Part model, mm, in its own coordinate system. Round coordinates to 2 decimals unless told otherwise and drop trailing zeros. Write each loop counter-clockwise with the first axis right and the second up, starting at its lowest first coordinate (ties: lowest second). Pieces come first, ordered by that corner, then holes. Notation, with made-up numbers: M 24,65 L 82,65 A22 cw 82,99 Z; hole C -35.5,-30.75 d11. An arc over 180 degrees is marked long. Use one line per item in the form item = value. Start each with the question number.
Item 1: Cut at A-A, the plane x = -29. Give the cut face in (y, z).
Item 2: Probe L1, parallel to X at y = -6.25, z = 24.5; L2, parallel to X at y = -11.25, z = -23.5. List the from-to ranges inside material, lowest first.
Item 3: Cut at B-B, the plane z = 24.5. Give the cut face in (x, y), then the cut area to 3 significant figures.
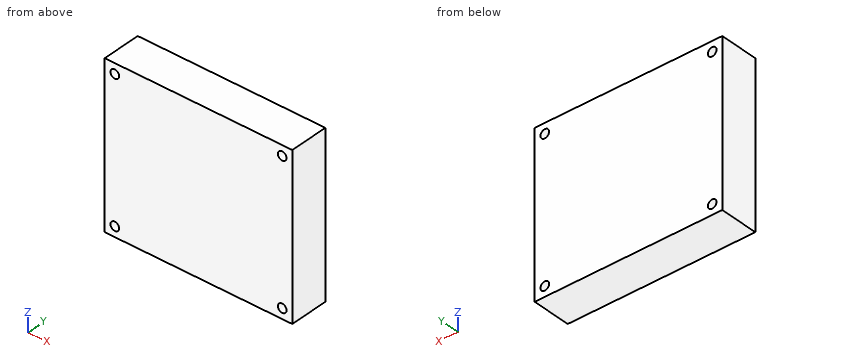
from build123d import *

# Parameters (mm, degrees)
SKETCH1_W           = 65
SKETCH1_H           = 56
BOSS_EXTRUDE1_DEPTH = 13.4
CUT_EXTRUDE1_REACH  = 46.942
SKETCH2_R           = 1.5


with BuildPart() as part:
    # Sketch1 → Boss-Extrude1 (new body)
    with BuildSketch(Plane(origin=(0, 0, 0), x_dir=(1, 0, 0), z_dir=(0, 1, 0))):
        Rectangle(SKETCH1_W, SKETCH1_H)
    extrude(amount=-BOSS_EXTRUDE1_DEPTH)

    # Sketch2 → Cut-Extrude1 (cut, up to next)
    with BuildSketch(Plane(origin=(0, 0, 0), x_dir=(1, 0, 0), z_dir=(0, 1, 0)), mode=Mode.PRIVATE) as cut_extrude1_sk1:
        with Locations(Location((29, 24.5, 0), (0, 0, 270))):
            Circle(SKETCH2_R)
    cut_extrude1_tool1 = extrude(cut_extrude1_sk1.sketch, amount=-CUT_EXTRUDE1_REACH, mode=Mode.PRIVATE) & part.part
    # Sketch2 → Cut-Extrude1 (cut, up to next)
    with BuildSketch(Plane(origin=(0, 0, 0), x_dir=(1, 0, 0), z_dir=(0, 1, 0)), mode=Mode.PRIVATE) as cut_extrude1_sk2:
        with Locations(Location((29, -24.5, 0), (0, 0, 270))):
            Circle(SKETCH2_R)
    cut_extrude1_tool2 = extrude(cut_extrude1_sk2.sketch, amount=-CUT_EXTRUDE1_REACH, mode=Mode.PRIVATE) & part.part
    # Sketch2 → Cut-Extrude1 (cut, up to next)
    with BuildSketch(Plane(origin=(0, 0, 0), x_dir=(1, 0, 0), z_dir=(0, 1, 0)), mode=Mode.PRIVATE) as cut_extrude1_sk3:
        with Locations(Location((-29, -24.5, 0), (0, 0, 270))):
            Circle(SKETCH2_R)
    cut_extrude1_tool3 = extrude(cut_extrude1_sk3.sketch, amount=-CUT_EXTRUDE1_REACH, mode=Mode.PRIVATE) & part.part
    # Sketch2 → Cut-Extrude1 (cut, up to next)
    with BuildSketch(Plane(origin=(0, 0, 0), x_dir=(1, 0, 0), z_dir=(0, 1, 0)), mode=Mode.PRIVATE) as cut_extrude1_sk4:
        with Locations(Location((-29, 24.5, 0), (0, 0, 270))):
            Circle(SKETCH2_R)
    cut_extrude1_tool4 = extrude(cut_extrude1_sk4.sketch, amount=-CUT_EXTRUDE1_REACH, mode=Mode.PRIVATE) & part.part
    add(cut_extrude1_tool1.solids().sort_by_distance((29, 0, -24.5))[0], mode=Mode.SUBTRACT)
    add(cut_extrude1_tool2.solids().sort_by_distance((29, 0, 24.5))[0], mode=Mode.SUBTRACT)
    add(cut_extrude1_tool3.solids().sort_by_distance((-29, 0, 24.5))[0], mode=Mode.SUBTRACT)
    add(cut_extrude1_tool4.solids().sort_by_distance((-29, 0, -24.5))[0], mode=Mode.SUBTRACT)


solid = part.part
Model answer:
q1.outline = M -13.4,-28 L 0,-28 L 0,-26 L -13.4,-26 Z; M -13.4,-23 L 0,-23 L 0,23 L -13.4,23 Z; M -13.4,26 L 0,26 L 0,28 L -13.4,28 Z
q2.L1 = -32.5 to -30.5, -27.5 to 27.5, 30.5 to 32.5
q2.L2 = -32.5 to -30.12, -27.88 to 27.88, 30.12 to 32.5
q3.outline = M -32.5,-13.4 L -30.5,-13.4 L -30.5,0 L -32.5,0 Z; M -27.5,-13.4 L 27.5,-13.4 L 27.5,0 L -27.5,0 Z; M 30.5,-13.4 L 32.5,-13.4 L 32.5,0 L 30.5,0 Z
q3.area = 791 mm²
